```python
from build123d import *

# Parameters (mm, degrees)
STOCK_AXIS_MASTER_1_START       = 135
STOCK_AXIS_MASTER_1_OUTLINE_R   = 1.5
STOCK_AXIS_MASTER_1_DEPTH       = 48
STOCK_AXIS_MASTER_1_START_2     = 185.5
STOCK_AXIS_MASTER_1_2_OUTLINE_R = 7.25
STOCK_AXIS_MASTER_1_2_DEPTH     = 19
STOCK_AXIS_MASTER_1_START_3     = 183
STOCK_AXIS_MASTER_1_3_OUTLINE_R = 11
STOCK_AXIS_MASTER_1_3_DEPTH     = 2
STOCK_AXIS_MASTER_1_START_4     = 185
STOCK_AXIS_MASTER_1_4_OUTLINE_R = 2.5
STOCK_AXIS_MASTER_1_4_DEPTH     = 22
CUT_EXTRUDE1_START              = -22
SKETCH1_R                       = 7.25
SKETCH1_R_2                     = 2.5
CUT_EXTRUDE1_DEPTH              = 22


# Read off the part's stored shape, not the designer's step: Stock-axis-master-1
with BuildPart() as part:
    # Stock-axis-master-1 outline → Stock-axis-master-1 (new body)
    with BuildSketch(Plane.YZ.offset(STOCK_AXIS_MASTER_1_START)):
        Polygon((49, -21), (52, -18), (52, 18), (49, 21), (13, 21), (10, 18), (10, -18), (13, -21), align=None)
        with Locations((15.5, -15.5)):
            Circle(STOCK_AXIS_MASTER_1_OUTLINE_R, mode=Mode.SUBTRACT)
        with Locations((46.5, -15.5)):
            Circle(STOCK_AXIS_MASTER_1_OUTLINE_R, mode=Mode.SUBTRACT)
        with Locations((15.5, 15.5)):
            Circle(STOCK_AXIS_MASTER_1_OUTLINE_R, mode=Mode.SUBTRACT)
        with Locations((46.5, 15.5)):
            Circle(STOCK_AXIS_MASTER_1_OUTLINE_R, mode=Mode.SUBTRACT)
    extrude(amount=STOCK_AXIS_MASTER_1_DEPTH)

    # Stock-axis-master-1 3 outline → Stock-axis-master-1 3 (add)
    with BuildSketch(Plane.YZ.offset(STOCK_AXIS_MASTER_1_START_3)):
        with Locations((31, 0)):
            Circle(STOCK_AXIS_MASTER_1_3_OUTLINE_R)
    extrude(amount=STOCK_AXIS_MASTER_1_3_DEPTH)



with BuildPart() as body_2:
    # Stock-axis-master-1 2 outline → Stock-axis-master-1 2 (new body)
    with BuildSketch(Plane.YZ.offset(STOCK_AXIS_MASTER_1_START_2)):
        with Locations((31, 0)):
            Circle(STOCK_AXIS_MASTER_1_2_OUTLINE_R)
    extrude(amount=STOCK_AXIS_MASTER_1_2_DEPTH)


with BuildPart() as part_1:
    add(part.part)

    add(body_2.part)  # Stock-axis-master-1 4 merges body 2
    # Stock-axis-master-1 4 outline → Stock-axis-master-1 4 (add)
    with BuildSketch(Plane.YZ.offset(STOCK_AXIS_MASTER_1_START_4)):
        with Locations((31, 0)):
            Circle(STOCK_AXIS_MASTER_1_4_OUTLINE_R)
    extrude(amount=STOCK_AXIS_MASTER_1_4_DEPTH)

    # Sketch1 → Cut-Extrude1 (cut)
    with BuildSketch(Plane(origin=(207, 0, 0), x_dir=(0, 0, -1), z_dir=(1, 0, 0)).offset(CUT_EXTRUDE1_START)):
        with Locations((0, 31)):
            Circle(SKETCH1_R)
        with Locations((0, 31)):
            Circle(SKETCH1_R_2, mode=Mode.SUBTRACT)
    extrude(amount=CUT_EXTRUDE1_DEPTH, mode=Mode.SUBTRACT)


solid = part_1.part
```
Work out the finished part from the listing and answer in its coordinate system (mm). A direction names the side the tool comes from. Coordinates: 2 decimals unless noted, no trailing zeros. Loops run counter-clockwise (first coordinate to the right, second up) from the corner with the lowest first, then second, coordinate; pieces in that order, holes last. Notation, with made-up numbers: M 39.25,31.5 L 51.25,31.5 A21 ccw 51.25,62.5 Z; hole C 16,34.25 d9. An arc over 180 degrees is marked long. Use CSV: the item, a comma, the result in double quotes. Start each with the question number.
(1) Find section A-A, the plane z = -15.5. Give the vertices of the cut face in (x, y).
(2) For faces 1 (the face through (183, 21, -9)), 2 (the face through (159, 31, 21)), determine the directions among +Z, -Z, +X, -X, +Y, -Y from which every point of the face is accessible in a straight line to the end or side of a thin tool.
(3) Find section B-B, the plane y = 46.5. Give the vertices of the cut face in (x, z).
(4) Find section C-C, the plane x = 170. Give the vertices of the cut face in (y, z).
(5) Consider line 1 (Z direction, x = 146.5, y = 15.5); line 2 (Y direction, x = 160.5, z = -15); line 3 (Z direction, x = 170, y = 46). Determine where each line is inside the solid, lowest interval first.
(6) Find section D-D, the plane z = -9. Give the vertices of the cut face in (x, y), then the cut area to 3 significant figures.
(7) Given pin 1 Ø5 at (y, z) = (15.5, -15.5) entering from +X; pin 2 Ø8 at (y, z) = (36, -7) entering from +X; pin 3 Ø5 at (y, z) = (46.5, -15.5) entering from -X; pin 4 Ø10 at (x, y) = (194, 40.5) entering from -Z, each flat-ended and moving along its own axis, determine where each tip first touches the part or whether it passes through.
Recorded:
1,outline,"M 135,10 L 183,10 L 183,14 L 135,14 Z; M 135,17 L 183,17 L 183,45 L 135,45 Z; M 135,48 L 183,48 L 183,52 L 135,52 Z"
2,face 1,"+X"
2,face 2,"+Z, +X, -X, +Y, -Y"
3,outline,"M 135,-21 L 183,-21 L 183,-17 L 135,-17 Z; M 135,-14 L 183,-14 L 183,14 L 135,14 Z; M 135,17 L 183,17 L 183,21 L 135,21 Z"
4,outline,"M 10,-18 L 13,-21 L 49,-21 L 52,-18 L 52,18 L 49,21 L 13,21 L 10,18 Z; hole C 15.5,-15.5 d3; hole C 15.5,15.5 d3; hole C 46.5,-15.5 d3; hole C 46.5,15.5 d3"
5,line 1,"z = -21 to -17, -14 to 14, 17 to 21"
5,line 2,"y = 10 to 14.09, 16.91 to 45.09, 47.91 to 52"
5,line 3,"z = -21 to -16.91, -14.09 to 14.09, 16.91 to 21"
6,outline,"M 135,10 L 183,10 L 183,24.68 L 185,24.68 L 185,37.32 L 183,37.32 L 183,52 L 135,52 Z"
6,area,"2,040 mm^2"
7,pin 1,"stops at x = 183"
7,pin 2,"stops at x = 185"
7,pin 3,"stops at x = 135"
7,pin 4,"passes through"
